Build history of the part. All positions in model axes, mm. Face numbers are marked on the shaded views. A direction names the side the tool comes from. Coordinates: 2 decimals unless noted, no trailing zeros. Order: outer loops, then holes, each group sorted by start corner. A loop starts at its lowest first (then second) coordinate and runs counter-clockwise, first axis right, second up. Notation, with made-up numbers: M 71.25,21 L 80.25,21 A17 cw 80.25,48 Z; hole C -23,-12 d7. An arc over 180 degrees is marked long. Use a Markdown table: item, result. Add a question column.
from build123d import *

# Parameters (mm, degrees)
CYLINDER016_R             = 3.25
CYLINDER016_DEPTH         = 12
CYLINDER015_R             = 4.25
CYLINDER015_DEPTH         = 15
CYLINDER017_R             = 2.75
CYLINDER017_DEPTH         = 48
FUSION004_PLACEMENT_ANGLE = 180


with BuildPart() as taladro001:
    # Cylinder016 → Cylinder016 (new body)
    with BuildSketch(Plane.XY):
        Circle(CYLINDER016_R)
    extrude(amount=CYLINDER016_DEPTH)


with BuildPart() as cilindro_exterior001:
    # Cylinder015 → Cylinder015 (new body)
    with BuildSketch(Plane.XY):
        Circle(CYLINDER015_R)
    extrude(amount=CYLINDER015_DEPTH)

    # Cut005: cut taladro001
    add(taladro001.part, mode=Mode.SUBTRACT)


with BuildPart() as fusion004:
    # Cylinder017 → Cylinder017 (new body)
    with BuildSketch(Plane.XY.offset(15)):
        Circle(CYLINDER017_R)
    extrude(amount=CYLINDER017_DEPTH)

    # Fusion004: union Cilindro exterior001
    add(cilindro_exterior001.part)


with BuildPart() as fusion004_1:
    # Fusion004 placement: moved
    add(fusion004.part.moved(Location((41, 167, 52))).rotate(Axis((41, 167, 52), (1, 0, 0)), FUSION004_PLACEMENT_ANGLE))


solid = fusion004_1.part
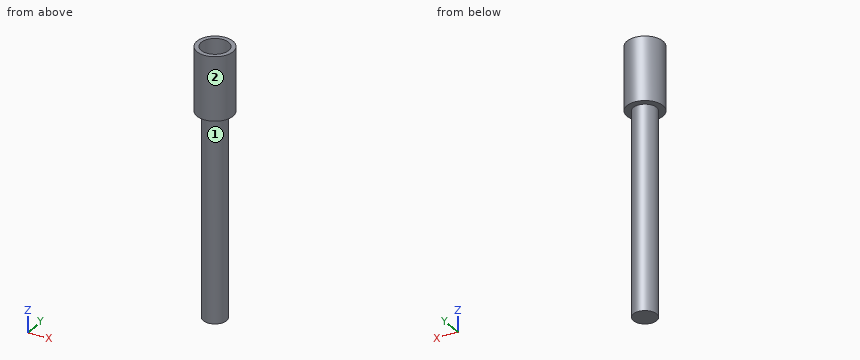
(1) Drop flat-ended pins along their axis: P1, Ø2, axis at x = 42.5, y = 166.5, coming from the +Z side; P2, Ø4, axis at y = 165.5, z = 22.5, coming from the -X side; P3, Ø1.5, axis at x = 38.5, z = -4.5, coming from the -Y side. Give the stop position or say it passes through.
(2) Drill centre lines: line 1 along X through (y, z) = (167, 45.25); line 2 along Y through (x, z) = (41, 43.75); line 3 along Z through (x, y) = (41, 168). Where is each one in solid material? Low to high. Write a range as from..to.
(3) Which spindle directions (+Z, -Z, +X, -X, +Y, -Y) get a long thin tool onto all of the face, cutting with end or side? Do the marked faces 1 and 2. Say none if no direction does.
(4) Slice it at D-D on z = -3.5. Give the cut face in (x, y), and give its area (3 significant figures).
(5) Slice it at A-A on y = 167. Give the cut face in (x, z), and give its area (4 significant figures).
(6) Slice it at C-C on z = 45. Give the cut face in (x, y).
(7) Slice it at B-B on x = 41. Give the cut face in (y, z).
Solutions:
| question | item | result |
|---|---|---|
| 1 | P1 | z = 40 |
| 1 | P2 | x = 38.25 |
| 1 | P3 | y = 164.88 |
| 2 | line 1 | 36.75..37.75, 44.25..45.25 |
| 2 | line 2 | 162.75..163.75, 170.25..171.25 |
| 2 | line 3 | -11..40 |
| 3 | face 1 | -Z |
| 3 | face 2 | +Z, -Z |
| 4 | outline | C 41,167 d5.5 |
| 4 | area | 23.8 mm² |
| 5 | outline | M 36.75,37 L 38.25,37 L 38.25,-11 L 43.75,-11 L 43.75,37 L 45.25,37 L 45.25,52 L 44.25,52 L 44.25,40 L 37.75,40 L 37.75,52 L 36.75,52 Z |
| 5 | area | 313.5 mm² |
| 6 | outline | C 41,167 d8.5; hole C 41,167 d6.5 |
| 7 | outline | M 162.75,37 L 164.25,37 L 164.25,-11 L 169.75,-11 L 169.75,37 L 171.25,37 L 171.25,52 L 170.25,52 L 170.25,40 L 163.75,40 L 163.75,52 L 162.75,52 Z |
